```python
from build123d import *

# Parameters (mm, degrees)
SKETCH1_W            = 120
SKETCH1_H            = 85
BOSS_EXTRUDE1_DEPTH  = 15
SKETCH9_W            = 12
SKETCH9_H            = 60
BOSS_EXTRUDE2_DEPTH  = 11
SKETCH10_W           = 76
SKETCH10_H           = 60
BOSS_EXTRUDE4_DEPTH  = 10
SKETCH12_W           = 3
SKETCH12_H           = 60
BOSS_EXTRUDE11_DEPTH = 6
BOSS_EXTRUDE12_DEPTH = 5
SKETCH14_W           = 76
SKETCH14_H           = 3
BOSS_EXTRUDE13_DEPTH = 8
SKETCH15_W           = 3
SKETCH15_H           = 15
SKETCH15_W_2         = 10
SKETCH15_H_2         = 7
BOSS_EXTRUDE14_DEPTH = 13
SKETCH16_W           = 120
SKETCH16_H           = 85
CUT_EXTRUDE3_DEPTH   = 4


with BuildPart() as part:
    # Sketch1 → Boss-Extrude1 (new body)
    with BuildSketch(Plane(origin=(0, 0, 0), x_dir=(1, 0, 0), z_dir=(0, 1, 0))):
        Rectangle(SKETCH1_W, SKETCH1_H)
        Polygon((-50, -30), (-53, -30), (-53, -7.5), (-56, -7.5), (-56, 7.5), (-53, 7.5), (-53, 25), (-53, 30), (-50, 30), (-38, 30), (-38, 33), (-5, 33), (-5, 40), (5, 40), (5, 33), (38, 33), (38, 30), (50, 30), (53, 30), (53, 7.5), (56, 7.5), (56, -7.5), (53, -7.5), (53, -30), (50, -30), (38, -30), (38, -33), (5, -33), (5, -40), (-5, -40), (-5, -33), (-38, -33), (-38, -30), align=None, mode=Mode.SUBTRACT)
    extrude(amount=BOSS_EXTRUDE1_DEPTH)

    # Sketch9 → Boss-Extrude2 (add)
    with BuildSketch(Plane(origin=(0, 0, 0), x_dir=(1, 0, 0), z_dir=(0, 1, 0))):
        with Locations((-44, 0)):
            Rectangle(SKETCH9_W, SKETCH9_H)
        with Locations((44, 0)):
            Rectangle(SKETCH9_W, SKETCH9_H)
    extrude(amount=BOSS_EXTRUDE2_DEPTH)

    # Sketch10 → Boss-Extrude4 (add)
    with BuildSketch(Plane(origin=(0, 0, 0), x_dir=(1, 0, 0), z_dir=(0, 1, 0))):
        Rectangle(SKETCH10_W, SKETCH10_H)
    extrude(amount=BOSS_EXTRUDE4_DEPTH)

    # Sketch12 → Boss-Extrude11 (add)
    with BuildSketch(Plane(origin=(0, 0, 0), x_dir=(1, 0, 0), z_dir=(0, 1, 0))):
        with Locations((-51.5, 0)):
            Rectangle(SKETCH12_W, SKETCH12_H)
        with Locations((51.5, 0)):
            Rectangle(SKETCH12_W, SKETCH12_H)
    extrude(amount=BOSS_EXTRUDE11_DEPTH)

    # Sketch13 → Boss-Extrude12 (add)
    with BuildSketch(Plane(origin=(0, 10, 0), x_dir=(1, 0, 0), z_dir=(0, 1, 0))):
        Polygon((-33, 19.981759626), (-33, 4), (-11.904077294, 4), align=None)
        Polygon((-26.375922706, 25), (-4, 8.048543405), (-4, 25), align=None)
        Polygon((4, 25), (4, 8.048543405), (26.375922706, 25), align=None)
        Polygon((11.904077294, 4), (33, 4), (33, 19.981759626), align=None)
        Polygon((11.904077294, -4), (33, -19.981759626), (33, -4), align=None)
        Polygon((4, -8.048543405), (4, -25), (26.375922706, -25), align=None)
        Polygon((-26.375922706, -25), (-4, -25), (-4, -8.048543405), align=None)
        Polygon((-33, -4), (-33, -19.981759626), (-11.904077294, -4), align=None)
    extrude(amount=BOSS_EXTRUDE12_DEPTH)

    # Sketch14 → Boss-Extrude13 (add)
    with BuildSketch(Plane(origin=(0, 0, 0), x_dir=(1, 0, 0), z_dir=(0, 1, 0))):
        with Locations((0, 31.5)):
            Rectangle(SKETCH14_W, SKETCH14_H)
        with Locations((0, -31.5)):
            Rectangle(SKETCH14_W, SKETCH14_H)
    extrude(amount=BOSS_EXTRUDE13_DEPTH)

    # Sketch15 → Boss-Extrude14 (add)
    with BuildSketch(Plane(origin=(0, 0, 0), x_dir=(1, 0, 0), z_dir=(0, 1, 0))):
        with Locations((-54.5, 0)):
            Rectangle(SKETCH15_W, SKETCH15_H)
        with Locations((0, -36.5)):
            Rectangle(SKETCH15_W_2, SKETCH15_H_2)
        with Locations((54.5, 0)):
            Rectangle(SKETCH15_W, SKETCH15_H)
        with Locations((0, 36.5)):
            Rectangle(SKETCH15_W_2, SKETCH15_H_2)
    extrude(amount=BOSS_EXTRUDE14_DEPTH)

    # Sketch16 → Cut-Extrude3 (cut)
    with BuildSketch(Plane.XZ):
        Rectangle(SKETCH16_W, SKETCH16_H)
    extrude(amount=-CUT_EXTRUDE3_DEPTH, mode=Mode.SUBTRACT)


solid = part.part
```
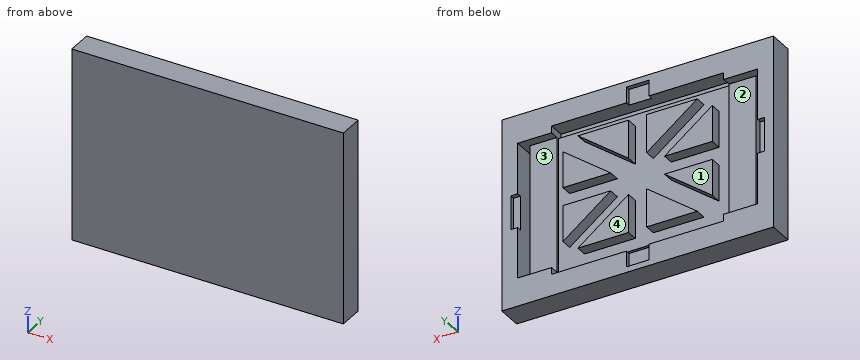
Here's how the part is built. I have some questions about the finished solid (model axes, mm). Face numbers are marked on the shaded views. A direction names the side the tool comes from. Coordinates: 2 decimals unless noted, no trailing zeros. Loops run counter-clockwise (first coordinate to the right, second up) from the corner with the lowest first, then second, coordinate; pieces in that order, holes last. Notation, with made-up numbers: (66.25, -14.5) -> (92.25, -14.5) arc R16 ccw to (92.25, 4.5) -> close; hole circle Ø4 at (9.25, 15.25). An arc over 180 degrees is marked (long way). Return JSON: item names as keys, results as strings.
1) For the marked faces 1 and 2, which set-ups out of +Z, -Z, +X, -X, +Y, -Y let a thin tool reach every point of the face, with its end or its side?
Results below:
{"face 1": "+Z, -Z, +X, -X, +Y", "face 2": "+Y"}
2) I need wall thicknesses on line 1 (X direction, y = 8.5, z = -4); line 2 (Z direction, x = -36.5, y = 13.25); line 3 (Z direction, x = 26, y = 8.5). Which ranges of each line are inside material? Lowest first, please. Write a range as from..to.
Results below:
{"line 1": "-60..-53, -50..50, 53..60", "line 2": "-42.5..-33, 33..42.5", "line 3": "-42.5..-33, -30..30, 33..42.5"}
3) Thinking about a two-plate mould opening in X: for the marked faces 3 and 4, which applies, +X half, -X half, draft (parallel to the pull), parting line (faces both ways), or undercut?
Results below:
{"face 3": "undercut", "face 4": "draft"}
4) If we section it at A-A, the plane z = 28.5: Write out the boundary of the cut face in (x, y).
Results below:
{"outline": "(-60, 4) -> (60, 4) -> (60, 15) -> (53, 15) -> (53, 6) -> (50, 6) -> (50, 11) -> (38, 11) -> (38, 10) -> (-38, 10) -> (-38, 11) -> (-50, 11) -> (-50, 6) -> (-53, 6) -> (-53, 15) -> (-60, 15) -> close"}
5) If we section it at C-C, the plane z = 2: Write out the boundary of the cut face in (x, y), then the cut area to 3 significant figures.
Results below:
{"outline": "(-60, 4) -> (60, 4) -> (60, 15) -> (56, 15) -> (56, 13) -> (53, 13) -> (53, 6) -> (50, 6) -> (50, 11) -> (38, 11) -> (38, 10) -> (-38, 10) -> (-38, 11) -> (-50, 11) -> (-50, 6) -> (-53, 6) -> (-53, 13) -> (-56, 13) -> (-56, 15) -> (-60, 15) -> close", "area": "778 mm²"}
6) If we section it at B-B, the plane x = -40: Write out the boundary of the cut face in (y, z), then the cut area to 3 significant figures.
Results below:
{"outline": "(4, -42.5) -> (15, -42.5) -> (15, -30) -> (11, -30) -> (11, 30) -> (15, 30) -> (15, 42.5) -> (4, 42.5) -> close", "area": "695 mm²"}
7) Will these pins go through, and if not, where does the flat tip stop? pin 1 (1.5 mm diameter, centred on x = 16.5, z = -31, fed in from +Y); pin 2 (2.5 mm diameter, centred on x = 51, z = -3.5, fed in from +Y); pin 3 (1.5 mm diameter, centred on x = -51.5, z = 10, fed in from +Y).
Results below:
{"pin 1": "y = 8", "pin 2": "y = 11", "pin 3": "y = 6"}
8) If we section it at D-D, the plane x = 19: Write out the boundary of the cut face in (y, z).
Results below:
{"outline": "(4, -42.5) -> (15, -42.5) -> (15, -33) -> (8, -33) -> (8, -30) -> (10, -30) -> (10, -25) -> (15, -25) -> (15, -19.41) -> (10, -19.41) -> (10, -9.38) -> (15, -9.38) -> (15, -4) -> (10, -4) -> (10, 4) -> (15, 4) -> (15, 9.38) -> (10, 9.38) -> (10, 19.41) -> (15, 19.41) -> (15, 25) -> (10, 25) -> (10, 30) -> (8, 30) -> (8, 33) -> (15, 33) -> (15, 42.5) -> (4, 42.5) -> close"}
